from build123d import *

# Parameters (mm, degrees)
SKETCH1_R           = 1.5
SKETCH1_W           = 6.096
SKETCH1_H           = 3
BOSS_EXTRUDE1_DEPTH = 1.499997


with BuildPart() as part:
    # Sketch1 → Boss-Extrude1 (new, symmetric)
    # profile 1 of 2: a face of its own
    with BuildSketch(Plane(origin=(0, 0, 0), x_dir=(0, 0, -1), z_dir=(1, 0, 0))):
        with BuildLine():
            ThreePointArc((8.69240433, -9.382807016), (8.888743448, -9.522527669), (9.093522628, -9.649556788))
            ThreePointArc((9.093522628, -9.649556788), (11.98462319, -10.030177398), (14.298079416, -8.255))
            Line((14.298079416, -8.255), (21.997045256, 5.08))
            Line((21.997045256, 5.08), (69.85, 5.08))
            Line((69.85, 5.08), (136.022177029, -61.092177029))
            Line((136.022177029, -61.092177029), (171.943201513, -25.171152545))
            Line((171.943201513, -25.171152545), (131.532048969, 15.24))
            Line((131.532048969, 15.24), (-19.050000183, 15.24))
            Line((-19.050000183, 15.24), (-19.050000183, 5.08))
            Line((-19.050000183, 5.08), (-7.332348419, 5.08))
            Line((-7.332348419, 5.08), (-3.299556755, -1.905000058))
            ThreePointArc((-3.299556755, -1.905000058), (-2.694076843, -2.694076843), (-1.905000058, -3.299556755))
            Line((-1.905000058, -3.299556755), (-0.860541922, -3.902574941))
            ThreePointArc((-0.860541922, -3.902574941), (0.874622108, -3.905666115), (2.448919028, -4.635318757))
            Line((2.448919028, -4.635318757), (8.69240433, -9.382807016))
        make_face()
        Polygon((137.442047446, -55.00257343), (135.320727102, -57.123893773), (131.010204164, -52.813370835), (133.131524508, -50.692050491), align=None, mode=Mode.SUBTRACT)
        Polygon((142.111780629, -51.7357401), (139.990460285, -49.614419757), (144.300983223, -45.303896819), (146.422303567, -47.425217162), align=None, mode=Mode.SUBTRACT)
        Polygon((128.461791325, -46.022317308), (126.340470981, -48.143637652), (122.029948043, -43.833114714), (124.151268387, -41.71179437), align=None, mode=Mode.SUBTRACT)
        Polygon((119.481535204, -37.042061187), (117.36021486, -39.163381531), (113.049691922, -34.852858593), (115.171012265, -32.731538249), align=None, mode=Mode.SUBTRACT)
        Polygon((110.501279083, -28.061805066), (108.379958739, -30.18312541), (104.069435801, -25.872602472), (106.190756144, -23.751282128), align=None, mode=Mode.SUBTRACT)
        Polygon((158.276241647, -35.571279083), (156.154921303, -33.449958739), (160.465444241, -29.139435801), (162.586764585, -31.260756144), align=None, mode=Mode.SUBTRACT)
        Polygon((167.974918257, -24.469702618), (165.853597914, -26.591022961), (161.543074976, -22.280500023), (163.664395319, -20.15917968), align=None, mode=Mode.SUBTRACT)
        Circle(SKETCH1_R, mode=Mode.SUBTRACT)
        with BuildLine():
            ThreePointArc((13.716146733, 3.67523044), (14.078517032, -1.85347193), (12.297560734, -7.1))
            ThreePointArc((12.297560734, -7.1), (10.248522628, -7.649038106), (9.699484522, -5.6))
            ThreePointArc((9.699484522, -5.6), (11.104182447, -1.461893353), (10.818369254, 2.898773305))
            ThreePointArc((10.818369254, 2.898773305), (11.879029426, 4.735890612), (13.716146733, 3.67523044))
        make_face(mode=Mode.SUBTRACT)
        with Locations((-12.700000556, 10.16)):
            Rectangle(SKETCH1_W, SKETCH1_H, mode=Mode.SUBTRACT)
        with Locations((-5.56e-07, 10.16)):
            Rectangle(SKETCH1_W, SKETCH1_H, mode=Mode.SUBTRACT)
        with Locations((12.699999444, 10.16)):
            Rectangle(SKETCH1_W, SKETCH1_H, mode=Mode.SUBTRACT)
        with Locations((25.399999444, 10.16)):
            Rectangle(SKETCH1_W, SKETCH1_H, mode=Mode.SUBTRACT)
        with Locations((38.099999444, 10.16)):
            Rectangle(SKETCH1_W, SKETCH1_H, mode=Mode.SUBTRACT)
        with Locations((50.799999444, 10.16)):
            Rectangle(SKETCH1_W, SKETCH1_H, mode=Mode.SUBTRACT)
        with Locations((63.499999444, 10.16)):
            Rectangle(SKETCH1_W, SKETCH1_H, mode=Mode.SUBTRACT)
        Polygon((101.521022961, -19.081548945), (99.399702618, -21.202869289), (95.08917968, -16.892346351), (97.210500023, -14.771026007), align=None, mode=Mode.SUBTRACT)
        Polygon((92.54076684, -10.101292824), (90.419446497, -12.222613168), (86.108923559, -7.91209023), (88.230243902, -5.790769886), align=None, mode=Mode.SUBTRACT)
        Polygon((158.994662136, -15.489446497), (156.873341793, -17.61076684), (152.562818855, -13.300243902), (154.684139198, -11.178923559), align=None, mode=Mode.SUBTRACT)
        Polygon((150.014406015, -6.509190376), (147.893085672, -8.630510719), (143.582562734, -4.319987781), (145.703883077, -2.198667438), align=None, mode=Mode.SUBTRACT)
        Polygon((83.560510719, -1.121036703), (81.439190376, -3.242357047), (77.128667438, 1.068165891), (79.249987781, 3.189486235), align=None, mode=Mode.SUBTRACT)
        Polygon((141.034149894, 2.471065745), (138.912829551, 0.349745402), (134.602306612, 4.66026834), (136.723626956, 6.781588683), align=None, mode=Mode.SUBTRACT)
    # profile 2 of 2: a face of its own
    with BuildSketch(Plane(origin=(0, 0, 0), x_dir=(0, 0, -1), z_dir=(1, 0, 0))):
        with BuildLine():
            ThreePointArc((-2.543703742, -4.709644618), (-1.749303433, -4.207713583), (-0.860541922, -3.902574941))
            Line((-0.860541922, -3.902574941), (-1.905000058, -3.299556755))
            ThreePointArc((-1.905000058, -3.299556755), (-2.694076843, -2.694076843), (-3.299556755, -1.905000058))
            Line((-3.299556755, -1.905000058), (-7.332348419, 5.08))
            Line((-7.332348419, 5.08), (-19.050000183, 5.08))
            Line((-19.050000183, 5.08), (-16.012126569, -4.882561423))
            ThreePointArc((-16.012126569, -4.882561423), (-15.354032248, -6.669430071), (-14.497265375, -8.370000042))
            ThreePointArc((-14.497265375, -8.370000042), (-11.736319841, -10.322059404), (-8.458544034, -9.491672897))
            Line((-8.458544034, -9.491672897), (-2.543703742, -4.709644618))
        make_face()
        with BuildLine():
            ThreePointArc((-12.297560842, -7.100000054), (-14.078517108, -1.853471934), (-13.716146726, 3.675230466))
            ThreePointArc((-13.716146726, 3.675230466), (-11.879029401, 4.735890605), (-10.818369261, 2.89877328))
            ThreePointArc((-10.818369261, 2.89877328), (-11.104182519, -1.461893392), (-9.699484623, -5.600000067))
            ThreePointArc((-9.699484623, -5.600000067), (-10.24852274, -7.64903817), (-12.297560842, -7.100000054))
        make_face(mode=Mode.SUBTRACT)
    extrude(amount=BOSS_EXTRUDE1_DEPTH, both=True)


solid = part.part
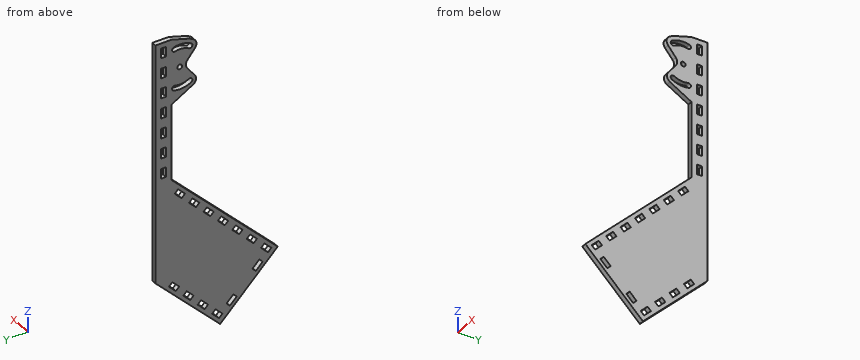
For this review, take the finished solid that the model builds, in its own axes (mm). Give positions to 0.01 mm unless a question says otherwise; leave off trailing zeros.
Item 1: Take a section at A-A, the plane x = -1. Give the number of separate pieces and of enclosed holes in the cut face, and give its area (3 significant figures).
Item 2: For line 1 along Y through (x, z) = (0.15, 0); line 2 along Z through (x, y) = (0.2, -24); line 3 along Z through (x, y) = (-0.75, -16), list the stretches that pass through material, from the lowest coordinate up.
Item 3: Insertion check: pin 1 (0.9 mm diameter, centred on x = 0.5, z = 12, fed in from -Y); pin 2 (0.9 mm diameter, centred on x = 0, y = 10, fed in from -Z); pin 3 (0.9 mm diameter, centred on x = 0.5, z = -47, fed in from -Y). Each pin has a flat end and moves straight along its axis. Give the tip position at first contact, or say it passes through.
Calculated:
1. separate pieces: 1
1. enclosed holes: 23
1. area: 5,050 mm2
2. line 1: y = -3.81 to -1.5, 1.5 to 8.66, 11.66 to 15.24
2. line 2: z = -170.77 to -167.51, -163.26 to -106.44, -105.94 to -98.93
2. line 3: z = -162.77 to -158.48, -155.26 to -98.44, -95.98 to -90.93
3. pin 1: stops at y = -10.35
3. pin 2: stops at z = -137.22
3. pin 3: stops at y = 5.08
